Work out the finished part from the listing and answer in its coordinate system (mm). A direction names the side the tool comes from. Give positions to 0.01 mm unless a question says otherwise; leave off trailing zeros. Answer as CSV lines item,"result". Start each with the question number.
1. For faces 1 (the flat face through (6.528, -4.74, 26.965)), 2 (the cylindrical face through (6.53, -7.83, -20.64)), 3 (the flat face through (6, -19, -25.4)), 4 (the flat face through (-6.35, -8, -24)), determine the directions among +Z, -Z, +X, -X, +Y, -Y from which every point of the face is accessible in a straight line to the end or side of a thin tool.
2. For a pull along Y with two mould halves and no side action, classify faces 5 (the cylindrical face through (57.664, -53.64, 7.968)), 6 (the flat face through (6, -2, -25.4)), 7 (the flat face through (6, -2, 25.4)) as released by +Y, released by -Y, zero draft, split by the parting line, or undercut.
3. Flat-ended cylindrical pins translate along their axes: pin 1 (3.5 mm diameter, centred on x = 9.5, y = -1.5, fed in from -Z); pin 2 (1.5 mm diameter, centred on x = 16, y = -7.5, fed in from +Z); pin 3 (23 mm diameter, centred on y = -7, z = 2, fed in from +X); pin 4 (10 mm diameter, centred on x = 33.5, z = 2.5, fed in from -Y). Find the tip coordinate at first contact, or state that the pin passes through.
4. Find the intervals of material crossed by L1, parallel to Y at x = 6.5, z = -17 (3 decimals); L2, parallel to Z at x = 9.5, y = -24; L3, parallel to Y at x = 3.5, z = -42 (3 decimals), in increasing order.
from build123d import *

# Parameters (mm, degrees)
SKETCH1_W                  = 38.1
SKETCH1_H                  = 50.8
BOSS_EXTRUDE1_DEPTH        = 3.175
SKETCH2_W                  = 38.1
SKETCH2_H                  = 19.05
BOSS_EXTRUDE2_DEPTH        = 28.575
SKETCH4_2_R                = 3.4925
IMAGINARYTUBING_DEPTH      = 12.7
IMAGINARYTUBING_DEPTH_BACK = 152.4
CUT_EXTRUDE1_DEPTH         = 12.7
SKETCH7_W                  = 25.4
SKETCH7_H                  = 9.525
BOSS_EXTRUDE4_DEPTH        = 3.175
BOSS_EXTRUDE5_DEPTH        = 25.4
CUT_EXTRUDE2_DEPTH         = 25.4


with BuildPart() as part:
    # Sketch1 → Boss-Extrude1 (new body)
    with BuildSketch(Plane(origin=(0, 0, 0), x_dir=(1, 0, 0), z_dir=(0, 1, 0))):
        Rectangle(SKETCH1_W, SKETCH1_H)
    extrude(amount=BOSS_EXTRUDE1_DEPTH)

    # Sketch2 → Boss-Extrude2 (add)
    with BuildSketch(Plane(origin=(0, 3.175, 0), x_dir=(1, 0, 0), z_dir=(0, 1, 0))):
        with Locations((0, 34.925)):
            Rectangle(SKETCH2_W, SKETCH2_H)
    extrude(amount=-BOSS_EXTRUDE2_DEPTH)

    # Sketch4<2> → ImaginaryTubing (add, two sides)
    with BuildSketch(Plane(origin=(-6.98065937, 6.98065937, -8.283711681), x_dir=(0.707106781, 0.707106781, 0), z_dir=(-0.54167522, 0.54167522, -0.64278761))) as imaginarytubing_sk:
        with Locations((0.967560903, 41.541493051)):
            Circle(SKETCH4_2_R)
    extrude(amount=IMAGINARYTUBING_DEPTH)
    extrude(imaginarytubing_sk.sketch, amount=-IMAGINARYTUBING_DEPTH_BACK)

    # Sketch6 → Cut-Extrude1 (cut)
    with BuildSketch(Plane.ZY.offset(19.05)):
        Polygon((-25.4, 0), (25.4, 0), (25.4, 3.175), (-44.45, 3.175), (-44.45, -25.4), (-25.4, -25.4), align=None)
    extrude(amount=-CUT_EXTRUDE1_DEPTH, mode=Mode.SUBTRACT)

    # Sketch7 → Boss-Extrude4 (add)
    with BuildSketch(Plane.XY.offset(25.4)):
        with Locations((6.35, -1.5875)):
            Rectangle(SKETCH7_W, SKETCH7_H)
    extrude(amount=BOSS_EXTRUDE4_DEPTH)

    # Sketch8 → Boss-Extrude5 (add)
    with BuildSketch(Plane(origin=(19.05, 0, 0), x_dir=(0, 0, -1), z_dir=(1, 0, 0))):
        with BuildLine():
            Line((25.4, -12.7), (25.4, -3.175))
            ThreePointArc((25.4, -3.175), (20.6375, -7.9375), (25.4, -12.7))
        make_face()
    extrude(amount=-BOSS_EXTRUDE5_DEPTH)

    # Sketch11 → Cut-Extrude2 (cut)
    with BuildSketch(Plane(origin=(19.05, 0, 0), x_dir=(0, 0, -1), z_dir=(1, 0, 0))):
        Polygon((-25.4, -3.175), (-28.575, -6.35), (-25.4, -6.35), align=None)
    extrude(amount=-CUT_EXTRUDE2_DEPTH, mode=Mode.SUBTRACT)


solid = part.part
Answer sheet:
1,face 1,"+X, -X, -Y"
1,face 2,"+X, -X"
1,face 3,"+Z, -X, -Y"
1,face 4,"+Z, -Z, -X, +Y, -Y"
2,face 5,"split by the parting line"
2,face 6,"undercut"
2,face 7,"zero draft"
3,pin 1,"stops at z = -49.64"
3,pin 2,"stops at z = -20.64"
3,pin 3,"stops at x = 19.05"
3,pin 4,"passes through"
4,L1,"y = 0 to 3.175"
4,L2,"z = -44.45 to -25.4"
4,L3,"y = -25.4 to 3.175"
